from build123d import *

# Parameters (mm, degrees)
SKETCH1_R               = 2.1
BOSS_EXTRUDE1_DEPTH     = 50
CUT_EXTRUDE1_DEPTH      = 77.342976101
CUT_EXTRUDE1_DEPTH_BACK = 77.342976101
SKETCH2_W               = 18.5
SKETCH2_H               = 12
SKETCH2_W_2             = 53
SKETCH2_H_2             = 46.5
SKETCH2_H_3             = 34.5
BOSS_EXTRUDE2_DEPTH     = 3.5
SKETCH4_R               = 2.08
CUT_EXTRUDE2_DEPTH      = 78.362781749


with BuildPart() as part:
    # Sketch1 → Boss-Extrude1 (new body)
    with BuildSketch(Plane(origin=(0, 0, 0), x_dir=(1, 0, 0), z_dir=(0, 1, 0))):
        with BuildLine():
            Line((22, 23.5), (-22, 23.5))
            ThreePointArc((-22, 23.5), (-24.828427125, 22.328427125), (-26, 19.5))
            Line((-26, 19.5), (-26, -47.5))
            ThreePointArc((-26, -47.5), (-24.828427125, -50.328427125), (-22, -51.5))
            Line((-22, -51.5), (22, -51.5))
            ThreePointArc((22, -51.5), (24.828427125, -50.328427125), (26, -47.5))
            Line((26, -47.5), (26, 19.5))
            ThreePointArc((26, 19.5), (24.828427125, 22.328427125), (22, 23.5))
        make_face()
        with Locations(Location((-12, -43, 0), (0, 0, 270))):
            Circle(SKETCH1_R, mode=Mode.SUBTRACT)
        with Locations(Location((12, -43, 0), (0, 0, 270))):
            Circle(SKETCH1_R, mode=Mode.SUBTRACT)
        with BuildLine():
            Line((11.5, 2.5), (11.5, -2.5))
            ThreePointArc((11.5, -2.5), (0, -14), (-11.5, -2.5))
            Line((-11.5, -2.5), (-11.5, 2.5))
            ThreePointArc((-11.5, 2.5), (0, 14), (11.5, 2.5))
        make_face(mode=Mode.SUBTRACT)
        with BuildLine():
            Line((-13.75, 18), (-13.75, 13))
            ThreePointArc((-13.75, 13), (-15.5, 11.25), (-17.25, 13))
            Line((-17.25, 13), (-17.25, 18))
            ThreePointArc((-17.25, 18), (-15.5, 19.75), (-13.75, 18))
        make_face(mode=Mode.SUBTRACT)
        with BuildLine():
            Line((17.25, 18), (17.25, 13))
            ThreePointArc((17.25, 13), (15.5, 11.25), (13.75, 13))
            Line((13.75, 13), (13.75, 18))
            ThreePointArc((13.75, 18), (15.5, 19.75), (17.25, 18))
        make_face(mode=Mode.SUBTRACT)
        with BuildLine():
            Line((17.25, -13), (17.25, -18))
            ThreePointArc((17.25, -18), (15.5, -19.75), (13.75, -18))
            Line((13.75, -18), (13.75, -13))
            ThreePointArc((13.75, -13), (15.5, -11.25), (17.25, -13))
        make_face(mode=Mode.SUBTRACT)
        with BuildLine():
            Line((-13.75, -13), (-13.75, -18))
            ThreePointArc((-13.75, -18), (-15.5, -19.75), (-17.25, -18))
            Line((-17.25, -18), (-17.25, -13))
            ThreePointArc((-17.25, -13), (-15.5, -11.25), (-13.75, -13))
        make_face(mode=Mode.SUBTRACT)
    extrude(amount=BOSS_EXTRUDE1_DEPTH)

    # Sketch2 → Cut-Extrude1 (cut, two sides: drawn at the far end of the back side and taken through both)
    with BuildSketch(Plane(origin=(0, 0, 0), x_dir=(0, 0, -1), z_dir=(1, 0, 0)).offset(-CUT_EXTRUDE1_DEPTH_BACK)):
        with Locations((-42.25, 44)):
            Rectangle(SKETCH2_W, SKETCH2_H)
        with Locations((-3, 23.25)):
            Rectangle(SKETCH2_W_2, SKETCH2_H_2)
        with Locations((-42.25, 17.25)):
            Rectangle(SKETCH2_W, SKETCH2_H_3)
    extrude(amount=CUT_EXTRUDE1_DEPTH + CUT_EXTRUDE1_DEPTH_BACK, mode=Mode.SUBTRACT)

    # Sketch3 → Boss-Extrude2 (add)
    with BuildSketch(Plane(origin=(26, 0, 0), x_dir=(0, 0, -1), z_dir=(1, 0, 0))):
        Polygon((19.5, 46.5), (-29.5, 0), (-29.5, 46.5), align=None)
        Polygon((-33, 50), (-47.5, 38), (-33, 38), align=None)
    boss_extrude2 = extrude(amount=-BOSS_EXTRUDE2_DEPTH)

    # Mirror1: Boss-Extrude2 across plane
    add(boss_extrude2.mirror(Plane(origin=(0, 0, 0), x_dir=(0, 0, 1), z_dir=(1, 0, 0))))

    # Sketch4 → Cut-Extrude2 (cut, through all)
    with BuildSketch(Plane(origin=(0, 0, 29.5), x_dir=(-1, 0, 0), z_dir=(0, 0, -1))):
        with Locations(Location((-12, 24.5, 0), (0, 0, 90))):
            Circle(SKETCH4_R)
        with Locations(Location((12, 24.5, 0), (0, 0, 90))):
            Circle(SKETCH4_R)
        with Locations(Location((0, 43.5, 0), (0, 0, 90))):
            Circle(SKETCH4_R)
    extrude(amount=-CUT_EXTRUDE2_DEPTH, mode=Mode.SUBTRACT)


solid = part.part
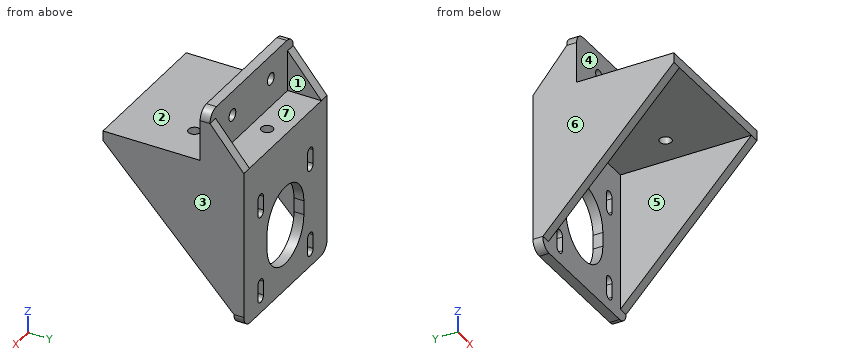
Verification items for the finished model (mm, model axes). Face numbers are marked on the shaded views. A direction names the side the tool comes from. Give positions to 0.01 mm unless a question says otherwise; leave off trailing zeros. Write each loop counter-clockwise with the first axis right and the second up, starting at its lowest first coordinate (ties: lowest second). Pieces come first, ordered by that corner, then holes. Notation, with made-up numbers: (12.25, 73) - (33.25, 73) arc R11 cw to (33.25, 85) - close; hole circle Ø6 at (58, -17). An arc over 180 degrees is marked (long way). Answer as CSV lines item,"result". Start each with the question number.
1. Thickness scan on line 1 (X direction, y = 36, z = 43); line 2 (Z direction, x = 12, y = 36.8); line 3 (X direction, y = 42, z = 33.5). Record the ranges inside material, lowest first.
2. Draft check along X on the marked faces 1, 2 and 3. Enter one of: pulls with the +X half, pulls with the -X half, needs draft (parallel to the pull), parting line crosses it, or undercut.
3. Sectioned sample at D-D (x = 8). Record the boundary of the cut face in (y, z), then the cut area to 3 significant figures.
4. Set-up check for the marked faces 4, 5, 6 and 7: record each of +Z, -Z, +X, -X, +Y, -Y from which the full face is reachable in a straight line by a thin tool's end or side.
5. Sectioned sample at B-B (y = 25). Record the boundary of the cut face in (x, z).
6. Depth check by flat-ended pin: pin 1 (1.5 mm diameter, centred on x = 20.5, z = -3.5, fed in from -Y); pin 2 (4 mm diameter, centred on x = -16.5, y = 25, fed in from +Z); pin 3 (14 mm diameter, centred on y = 13.5, z = 7.5, fed in from +X); pin 4 (9 mm diameter, centred on x = 1, z = 44, fed in from +Y). Enter the tip coordinate at first touch or a pass-through.
7. Sectioned sample at A-A (x = -15.5). Record the boundary of the cut face in (y, z).
8. Sectioned sample at C-C (z = -6). Record the boundary of the cut face in (x, y), then the cut area to 3 significant figures.
Derived:
1,line 1,"-26 to -14.1, -9.9 to 9.9, 14.1 to 26"
1,line 2,"29.5 to 40.9, 45.1 to 51.5"
1,line 3,"-26 to -22.5, 22.5 to 26"
2,face 1,"undercut"
2,face 2,"needs draft"
2,face 3,"pulls with the +X half"
3,outline,"(0, 29.5) - (46.5, 29.5) - (46.5, 10.76) - (50, 10.76) - (50, 33) - (38, 33) - (38, 51.5) - (34.5, 51.5) - (34.5, 33) - (0, 33) - close; (46.5, -23.5) - (50, -23.5) - (50, -10.76) - (46.5, -10.76) - close"
3,area,"350 mm²"
4,face 4,"+Z, +X, -X, -Y"
4,face 5,"-Z, -Y"
4,face 6,"+Z, -Z, -X, +Y, -Y"
4,face 7,"+Z, +Y"
5,outline,"(-26, 3.16) - (-22.5, 3.16) - (-22.5, 29.5) - (-14.02, 29.5) - (-14.02, 33) - (-26, 33) - close; (-9.98, 29.5) - (9.98, 29.5) - (9.98, 33) - (-9.98, 33) - close; (14.02, 29.5) - (22.5, 29.5) - (22.5, 3.16) - (26, 3.16) - (26, 33) - (14.02, 33) - close"
6,pin 1,"y = 46.5"
6,pin 2,"z = 33"
6,pin 3,"x = 26"
6,pin 4,"y = 38"
7,outline,"(0, 29.5) - (46.5, 29.5) - (46.5, 19.75) - (50, 19.75) - (50, 33) - (38, 33) - (38, 51.5) - (34.5, 51.5) - (34.5, 33) - (0, 33) - close; (46.5, -23.5) - (50, -23.5) - (50, -19.75) - (46.5, -19.75) - close; (46.5, -11.25) - (50, -11.25) - (50, 11.25) - (46.5, 11.25) - close"
8,outline,"(-26, 33.69) - (-22.5, 33.69) - (-22.5, 46.5) - (-10.95, 46.5) - (-10.95, 50) - (-26, 50) - close; (10.95, 46.5) - (22.5, 46.5) - (22.5, 33.69) - (26, 33.69) - (26, 50) - (10.95, 50) - close"
8,area,"195 mm²"
